CAD build for the part. Positions are in the model's coordinates, mm. Give positions to 0.01 mm unless a question says otherwise; leave off trailing zeros. Loops run counter-clockwise (first coordinate to the right, second up) from the corner with the lowest first, then second, coordinate; pieces in that order, holes last.
Item 1: Probe probe 1 along X at (y, z) = (-7.75, 0.4); probe 2 along Y at (x, z) = (0, 0.5); probe 3 along Y at (x, z) = (8, 1.1). List the from-to ranges inside material, lowest first.
Item 2: Saw through at B-B on x = 3.5. Give the cut face in (y, z), plus the area to 3 significant figures.
Item 3: Saw through at A-A on z = 1.3. Give the number of separate pieces and of enclosed holes in the cut face, plus the area to 3 significant figures.
Item 4: Mould opens along X. For faces 1 (the cylindrical face through (-0.54, -2.44, 0.99)), 2 (the flat face through (2, -2, 0)), 3 (the cylindrical face through (10, 3.2, 1)) say: released by +X, released by -X, zero draft, split by the parting line, or undercut.
Item 5: Saw through at C-C on x = -7.5. Give the cut face in (y, z).
from build123d import *

# Parameters (mm, degrees)
CROQUIS1_R              = 10.5
CROQUIS1_R_2            = 0.75
CROQUIS1_R_3            = 2.5
SALIENTE_EXTRUIR1_DEPTH = 2


with BuildPart() as part:
    # Croquis1 → Saliente-Extruir1 (new body)
    with BuildSketch(Plane.XY):
        Circle(CROQUIS1_R)
        with Locations((0, 7.5)):
            Circle(CROQUIS1_R_2, mode=Mode.SUBTRACT)
        with Locations((-3.5, 7.5)):
            Circle(CROQUIS1_R_2, mode=Mode.SUBTRACT)
        with Locations((3.5, 7.5)):
            Circle(CROQUIS1_R_2, mode=Mode.SUBTRACT)
        with Locations((7.5, 3.5)):
            Circle(CROQUIS1_R_2, mode=Mode.SUBTRACT)
        with Locations((7.5, 0)):
            Circle(CROQUIS1_R_2, mode=Mode.SUBTRACT)
        with Locations((7.5, -3.5)):
            Circle(CROQUIS1_R_2, mode=Mode.SUBTRACT)
        with Locations((3.5, -7.5)):
            Circle(CROQUIS1_R_2, mode=Mode.SUBTRACT)
        with Locations((0, -7.5)):
            Circle(CROQUIS1_R_2, mode=Mode.SUBTRACT)
        with Locations((-3.5, -7.5)):
            Circle(CROQUIS1_R_2, mode=Mode.SUBTRACT)
        with Locations((-7.5, -3.5)):
            Circle(CROQUIS1_R_2, mode=Mode.SUBTRACT)
        with Locations((-7.5, 0)):
            Circle(CROQUIS1_R_2, mode=Mode.SUBTRACT)
        with Locations((-7.5, 3.5)):
            Circle(CROQUIS1_R_2, mode=Mode.SUBTRACT)
        Circle(CROQUIS1_R_3, mode=Mode.SUBTRACT)
    extrude(amount=SALIENTE_EXTRUIR1_DEPTH)


solid = part.part
Results below:
1. probe 1: x = -7.08 to -4.21, -2.79 to -0.71, 0.71 to 2.79, 4.21 to 7.08
1. probe 2: y = -10.5 to -8.25, -6.75 to -2.5, 2.5 to 6.75, 8.25 to 10.5
1. probe 3: y = -6.8 to -4.06, -2.94 to -0.56, 0.56 to 2.94, 4.06 to 6.8
2. outline: (-9.9, 0) - (-8.25, 0) - (-8.25, 2) - (-9.9, 2) - close; (-6.75, 0) - (6.75, 0) - (6.75, 2) - (-6.75, 2) - close; (8.25, 0) - (9.9, 0) - (9.9, 2) - (8.25, 2) - close
2. area: 33.6 mm2
3. separate pieces: 1
3. enclosed holes: 13
3. area: 306 mm2
4. face 1: undercut
4. face 2: zero draft
4. face 3: split by the parting line
5. outline: (-7.35, 0) - (-4.25, 0) - (-4.25, 2) - (-7.35, 2) - close; (-2.75, 0) - (-0.75, 0) - (-0.75, 2) - (-2.75, 2) - close; (0.75, 0) - (2.75, 0) - (2.75, 2) - (0.75, 2) - close; (4.25, 0) - (7.35, 0) - (7.35, 2) - (4.25, 2) - close
